Source: CAD feature listing. Evaluate the final solid. Frame: model axes, mm. Face numbers are marked on the shaded views. A direction names the side the tool comes from. Coordinates: 2 decimals unless noted, no trailing zeros. Write each loop counter-clockwise with the first axis right and the second up, starting at its lowest first coordinate (ties: lowest second). Pieces come first, ordered by that corner, then holes. Notation, with made-up numbers: (-27, 58.5) - (10, 58.5) arc R34 cw to (10, 93.5) - close; hole circle Ø4 at (76, -29). An arc over 180 degrees is marked (long way). One line per item, written item: value.
from build123d import *

# Parameters (mm, degrees)
F0_W     = 169.640712
F0_H     = 92.04305
F0_W_2   = 157.417692
F0_H_2   = 77.59766
F1_DEPTH = 25.4
F2_R     = 2.452841
F3_R     = 2.4638


with BuildPart() as f1:
    # F0 (on Right) → F1 (new body)
    with BuildSketch(Plane.YZ):
        with Locations((-0.161145, -1.181595)):
            Rectangle(F0_W, F0_H)
        with Locations((0.024054, -1.366796)):
            Rectangle(F0_W_2, F0_H_2, mode=Mode.SUBTRACT)
    extrude(amount=F1_DEPTH)

    # F2
    f2_edges = [f1.edges().sort_by_distance(p)[0] for p in [
        (25.4, -0.161145, -47.20312),
        (25.4, -84.981501, -1.181595),
        (25.4, -0.161145, 44.83993),
        (25.4, 84.659211, -1.181595),
    ]]
    fillet(f2_edges, radius=F2_R)

    # F3
    f3_edges = [f1.edges().sort_by_distance(p)[0] for p in [
        (0, 84.659211, -1.181595),
        (0, -0.161145, 44.83993),
        (0, -0.161145, -47.20312),
        (0, -84.981501, -1.181595),
    ]]
    fillet(f3_edges, radius=F3_R)


solid = f1.part
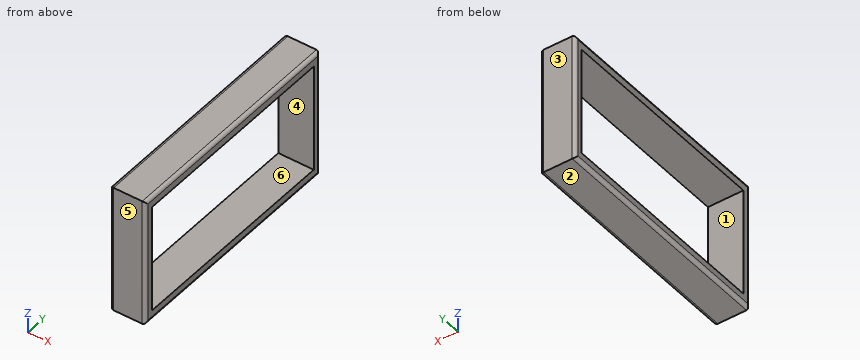
1) Section query B-B on z = 23. Output: boundary loops of the cut face in (x, y), then the cut area to 3 significant figures.
Values found:
outline: (0, -82.52) arc R2.46 ccw to (2.46, -84.98) - (22.95, -84.98) arc R2.45 ccw to (25.4, -82.53) - (25.4, -78.68) - (0, -78.68) - close; (0, 78.73) - (25.4, 78.73) - (25.4, 82.21) arc R2.45 ccw to (22.95, 84.66) - (2.46, 84.66) arc R2.46 ccw to (0, 82.2) - close
area: 305 mm2
2) Material intervals for line 1 (Z direction, x = 17.75, y = -36.5); line 2 (Y direction, x = 19.5, z = -30); line 3 (Y direction, x = 2, z = -26.5), sorted ascending.
Values found:
line 1: -47.2 to -40.17, 37.43 to 44.84
line 2: -84.98 to -78.68, 78.73 to 84.66
line 3: -84.94 to -78.68, 78.73 to 84.62
3) Section query A-A on y = 53. Output: boundary loops of the cut face in (x, z), then the cut area to 3 significant figures.
Values found:
outline: (0, -44.74) arc R2.46 ccw to (2.46, -47.2) - (22.95, -47.2) arc R2.45 ccw to (25.4, -44.75) - (25.4, -40.17) - (0, -40.17) - close; (0, 37.43) - (25.4, 37.43) - (25.4, 42.39) arc R2.45 ccw to (22.95, 44.84) - (2.46, 44.84) arc R2.46 ccw to (0, 42.38) - close
area: 362 mm2
4) Section query C-C on x = 10. Output: boundary loops of the cut face in (y, z).
Values found:
outline: (-84.98, -47.2) - (84.66, -47.2) - (84.66, 44.84) - (-84.98, 44.84) - close; hole (-78.68, -40.17) - (78.73, -40.17) - (78.73, 37.43) - (-78.68, 37.43) - close
5) Draft query along Y for the marked faces 1, 2, 3 and 4. Return one class per face: released by +Y, released by -Y, zero draft, split by the parting line, or undercut.
Values found:
face 1: undercut
face 2: zero draft
face 3: released by +Y
face 4: undercut
6) Reachability of the marked faces 5 and 6 from +Z, -Z, +X, -X, +Y, -Y: full face, straight path, thin tool, end or side. Return the list, or none.
Values found:
face 5: +Z, -Z, +X, -X, -Y
face 6: +X, -X
